from build123d import *

# Parameters (mm, degrees)
F0_R     = 5
F2_DEPTH = 12.5
F1_R     = 5
F3_DEPTH = 5


# Not quite as in the source:
# - a feature of the source that left no trace in its solid (it failed there, or was rolled back) is left out


with BuildPart() as f2:
    # F0 (on Top) → F2 (new body, symmetric)
    with BuildSketch(Plane.XY):
        with BuildLine():
            ThreePointArc((7.2403054276, -13.0434782609), (5.5090082779, 0), (7.2403054276, 13.0434782609))
            ThreePointArc((7.2403054276, 13.0434782609), (2.3044883911, 22.1371796429), (-7.0173413473, 17.6470588235))
            ThreePointArc((-7.0173413473, 17.6470588235), (-10.2350656985, 0), (-7.0173413473, -17.6470588235))
            ThreePointArc((-7.0173413473, -17.6470588235), (2.3044883911, -22.1371796429), (7.2403054276, -13.0434782609))
        make_face()
        with Locations((0, -15)):
            Circle(F0_R, mode=Mode.SUBTRACT)
        with Locations((0, 15)):
            Circle(F0_R, mode=Mode.SUBTRACT)
    extrude(amount=F2_DEPTH, both=True)

    # F1 (on Top) → F3 (join, symmetric)
    with BuildSketch(Plane.XY):
        with BuildLine():
            ThreePointArc((38.9229935461, 38.1714845638), (12.7620087728, 36.2695311392), (-6.5959822677, 18.5697363943))
            ThreePointArc((-6.5959822677, 18.5697363943), (-3.5697363943, 8.4040177323), (6.5959822677, 11.4302636057))
            ThreePointArc((6.5959822677, 11.4302636057), (15.785676778, 21.0076181762), (28.5825898266, 24.5311422915))
            Line((28.5825898266, 24.5311422915), (30.5825898266, 24.5311422915))
            Line((30.5825898266, 24.5311422915), (32.5825898266, 24.5311422915))
            Line((32.5825898266, 24.5311422915), (34.5825898266, 24.5311422915))
            Line((34.5825898266, 24.5311422915), (36.5825898266, 24.5311422915))
            Line((36.5825898266, 24.5311422915), (38.5825898266, 24.5311422915))
            Line((38.5825898266, 24.5311422915), (40.5825898266, 24.5311422915))
            Line((40.5825898266, 24.5311422915), (42.5825898266, 24.5311422915))
            Line((42.5825898266, 24.5311422915), (44.5825898266, 24.5311422915))
            Line((44.5825898266, 24.5311422915), (46.5825898266, 24.5311422915))
            Line((46.5825898266, 24.5311422915), (48.5825898266, 24.5311422915))
            Line((48.5825898266, 24.5311422915), (60, 32.5311422915))
            Line((60, 32.5311422915), (38.9229935461, 38.1714845638))
        make_face()
        with Locations((0, 15)):
            Circle(F1_R, mode=Mode.SUBTRACT)
        with BuildLine():
            ThreePointArc((22.4425128865, 31.74578129), (21.0275159589, 34.1948185896), (23.4765532585, 35.6098155172))
            Line((23.4765532585, 35.6098155172), (37.9666816106, 31.7321641224))
            ThreePointArc((37.9666816106, 31.7321641224), (39.0361733804, 31.017923595), (39.4496614246, 29.8001470088))
            ThreePointArc((39.4496614246, 29.8001470088), (38.6674380108, 28.2136350529), (36.9326412386, 27.8681298951))
            Line((36.9326412386, 27.8681298951), (22.4425128865, 31.74578129))
        make_face(mode=Mode.SUBTRACT)
        with BuildLine():
            Line((32.5825898266, -24.5311422915), (30.5825898266, -24.5311422915))
            Line((30.5825898266, -24.5311422915), (28.5825898266, -24.5311422915))
            ThreePointArc((28.5825898266, -24.5311422915), (15.785676778, -21.0076181762), (6.5959822677, -11.4302636057))
            ThreePointArc((6.5959822677, -11.4302636057), (-3.5697363943, -8.4040177323), (-6.5959822677, -18.5697363943))
            ThreePointArc((-6.5959822677, -18.5697363943), (12.7620087728, -36.2695311392), (38.9229935461, -38.1714845638))
            Line((38.9229935461, -38.1714845638), (60, -32.5311422915))
            Line((60, -32.5311422915), (48.5825898266, -24.5311422915))
            Line((48.5825898266, -24.5311422915), (46.5825898266, -24.5311422915))
            Line((46.5825898266, -24.5311422915), (44.5825898266, -24.5311422915))
            Line((44.5825898266, -24.5311422915), (42.5825898266, -24.5311422915))
            Line((42.5825898266, -24.5311422915), (40.5825898266, -24.5311422915))
            Line((40.5825898266, -24.5311422915), (38.5825898266, -24.5311422915))
            Line((38.5825898266, -24.5311422915), (36.5825898266, -24.5311422915))
            Line((36.5825898266, -24.5311422915), (34.5825898266, -24.5311422915))
            Line((34.5825898266, -24.5311422915), (32.5825898266, -24.5311422915))
        make_face()
        with Locations((0, -15)):
            Circle(F1_R, mode=Mode.SUBTRACT)
        with BuildLine():
            ThreePointArc((23.4765532585, -35.6098155172), (21.0275159589, -34.1948185896), (22.4425128865, -31.74578129))
            Line((22.4425128865, -31.74578129), (36.9326412386, -27.8681298951))
            ThreePointArc((36.9326412386, -27.8681298951), (38.6674380108, -28.2136350529), (39.4496614246, -29.8001470088))
            ThreePointArc((39.4496614246, -29.8001470088), (39.0361733804, -31.017923595), (37.9666816106, -31.7321641224))
            Line((37.9666816106, -31.7321641224), (23.4765532585, -35.6098155172))
        make_face(mode=Mode.SUBTRACT)
        Polygon((30.5825898266, 24.5311422915), (28.5825898266, 24.5311422915), (29.5825898266, 23.5311422915), align=None)
        Polygon((32.5825898266, 24.5311422915), (30.5825898266, 24.5311422915), (31.5825898266, 23.5311422915), align=None)
        Polygon((34.5825898266, 24.5311422915), (32.5825898266, 24.5311422915), (33.5825898266, 23.5311422915), align=None)
        Polygon((36.5825898266, 24.5311422915), (34.5825898266, 24.5311422915), (35.5825898266, 23.5311422915), align=None)
        Polygon((38.5825898266, 24.5311422915), (36.5825898266, 24.5311422915), (37.5825898266, 23.5311422915), align=None)
        Polygon((40.5825898266, 24.5311422915), (38.5825898266, 24.5311422915), (39.5825898266, 23.5311422915), align=None)
        Polygon((41.5825898266, 23.5311422915), (42.5825898266, 24.5311422915), (40.5825898266, 24.5311422915), align=None)
        Polygon((43.5825898266, 23.5311422915), (44.5825898266, 24.5311422915), (42.5825898266, 24.5311422915), align=None)
        Polygon((45.5825898266, 23.5311422915), (46.5825898266, 24.5311422915), (44.5825898266, 24.5311422915), align=None)
        Polygon((47.5825898266, 23.5311422915), (48.5825898266, 24.5311422915), (46.5825898266, 24.5311422915), align=None)
        Polygon((30.5825898266, -24.5311422915), (29.5825898266, -23.5311422915), (28.5825898266, -24.5311422915), align=None)
        Polygon((31.5825898266, -23.5311422915), (30.5825898266, -24.5311422915), (32.5825898266, -24.5311422915), align=None)
        Polygon((33.5825898266, -23.5311422915), (32.5825898266, -24.5311422915), (34.5825898266, -24.5311422915), align=None)
        Polygon((35.5825898266, -23.5311422915), (34.5825898266, -24.5311422915), (36.5825898266, -24.5311422915), align=None)
        Polygon((37.5825898266, -23.5311422915), (36.5825898266, -24.5311422915), (38.5825898266, -24.5311422915), align=None)
        Polygon((39.5825898266, -23.5311422915), (38.5825898266, -24.5311422915), (40.5825898266, -24.5311422915), align=None)
        Polygon((41.5825898266, -23.5311422915), (40.5825898266, -24.5311422915), (42.5825898266, -24.5311422915), align=None)
        Polygon((43.5825898266, -23.5311422915), (42.5825898266, -24.5311422915), (44.5825898266, -24.5311422915), align=None)
        Polygon((44.5825898266, -24.5311422915), (46.5825898266, -24.5311422915), (45.5825898266, -23.5311422915), align=None)
        Polygon((46.5825898266, -24.5311422915), (48.5825898266, -24.5311422915), (47.5825898266, -23.5311422915), align=None)
    extrude(amount=F3_DEPTH, both=True)


solid = f2.part
Geometry check sheet. Reference: the model listing, model coordinates, mm. A direction names the side the tool comes from. Give positions to 0.01 mm unless a question says otherwise; leave off trailing zeros. Write each loop counter-clockwise with the first axis right and the second up, starting at its lowest first coordinate (ties: lowest second). Pieces come first, ordered by that corner, then holes.
1) Release check for a two-part mould opening along X. For faces 3 (the face through (54.211, 28.475, -0.07)), 4 (the face through (21.04, -34.24, 0.07)), 5 (the face through (26, 29, 5)) record: released by +X, released by -X, zero draft, split by the parting line, or undercut.
Values follow:
face 3: released by +X
face 4: undercut
face 5: zero draft
2) Go/stop test with flat-tipped pins: pin 1 Ø4 at (y, z) = (15, 10) entering from +X; pin 2 Ø1 at (y, z) = (3, -9.5) entering from +X; pin 3 Ø4 at (x, y) = (10.5, -28.5) entering from +Z; pin 4 Ø22 at (x, y) = (12, 20) entering from +Z. Record where each tip stops, or that it passes through.
Values follow:
pin 1: stops at x = 7.5
pin 2: stops at x = 5.63
pin 3: stops at z = 5
pin 4: stops at z = 12.5
3) Cross-section at B-B (z = -6). Record the boundary of the cut face in (x, y), plus the area to 3 significant figures.
Values follow:
outline: (-7.02, -17.65) arc R7.5 ccw to (7.24, -13.04) arc R50 cw to (7.24, 13.04) arc R7.5 ccw to (-7.02, 17.65) arc R50 ccw to start; hole circle Ø10 at (0, -15); hole circle Ø10 at (0, 15)
area: 492 mm2
4) Thickness scan on line 1 (Y direction, x = 0, z = 6.5); line 2 (Y direction, x = 0, z = 1); line 3 (Z direction, x = 30.5, y = -25.5). Record the ranges inside material, lowest first.
Values follow:
line 1: y = -22.5 to -20, -10 to 10, 20 to 22.5
line 2: y = -27.51 to -20, -10 to 10, 20 to 27.51
line 3: z = -5 to 5
5) Cross-section at C-C (x = 0). Record the boundary of the cut face in (y, z), plus the area to 3 significant figures.
Values follow:
outline: (-27.51, -5) - (-22.5, -5) - (-22.5, -12.5) - (-20, -12.5) - (-20, 12.5) - (-22.5, 12.5) - (-22.5, 5) - (-27.51, 5) - close; (-10, -12.5) - (10, -12.5) - (10, 12.5) - (-10, 12.5) - close; (20, -12.5) - (22.5, -12.5) - (22.5, -5) - (27.51, -5) - (27.51, 5) - (22.5, 5) - (22.5, 12.5) - (20, 12.5) - close
area: 725 mm2
6) Set-up check for faces 1 (the face through (49.61, 35.31, -0.07)), 2 (the face through (30.823, -33.644, 0.07)): record each of +Z, -Z, +X, -X, +Y, -Y from which the full face is reachable in a straight line by a thin tool's end or side.
Values follow:
face 1: +Z, -Z, +X, +Y
face 2: +Z, -Z
7) Cross-section at D-D (y = 15). Record the boundary of the cut face in (x, z).
Values follow:
outline: (-7.93, -12.5) - (-5, -12.5) - (-5, 12.5) - (-7.93, 12.5) - close; (5, -12.5) - (7.5, -12.5) - (7.5, -5) - (8.94, -5) - (8.94, 5) - (7.5, 5) - (7.5, 12.5) - (5, 12.5) - close
8) Cross-section at A-A (x = 11). Record the boundary of the cut face in (y, z), plus the area to 3 significant figures.
Values follow:
outline: (-35.46, -5) - (-17.3, -5) - (-17.3, 5) - (-35.46, 5) - close; (17.3, -5) - (35.46, -5) - (35.46, 5) - (17.3, 5) - close
area: 363 mm2
